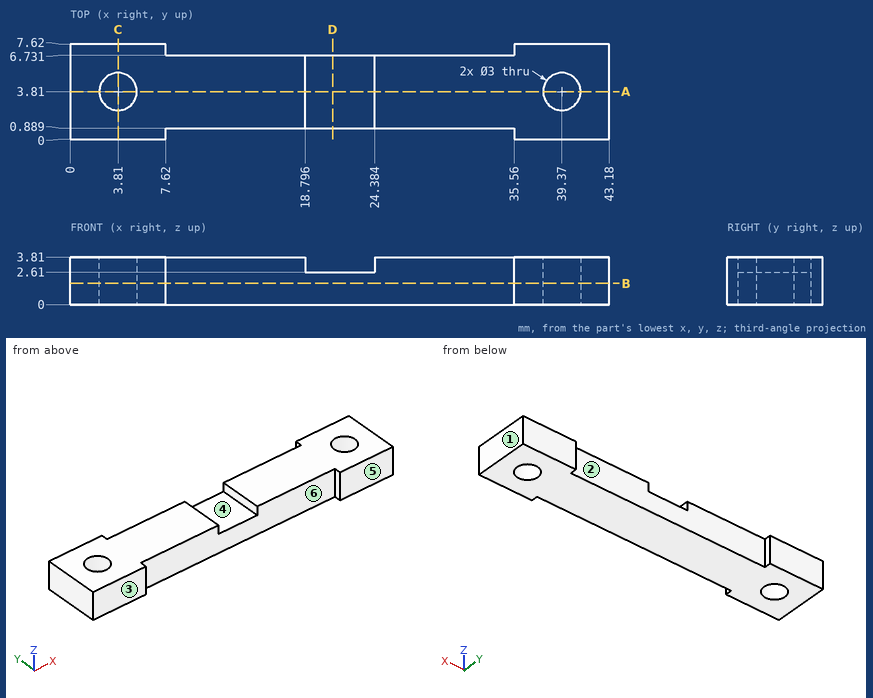
Answer from the drawing. Dimensions are ordinates in mm from the lowest x, y and z of the part. A direction names the side the tool comes from. Give positions to 0.01 mm unless a question says otherwise; leave off trailing zeros. Loops run counter-clockwise (first coordinate to the right, second up) from the corner with the lowest first, then second, coordinate; pieces in that order, holes last. Notation, with made-up numbers: (64, 80) - (96, 80) arc R20 ccw to (96, 113) - close; hole circle Ø7 at (86, 4). An arc over 180 degrees is marked (long way). Answer as CSV lines item,"result". Start each with the question number.
Item 1: Each of these flat-tipped pins is pushed along its axis until it touches: pin 1 (1.9 mm diameter, centred on x = 26, z = 1, fed in from +Y); pin 2 (2.5 mm diameter, centred on x = 3.81, y = 3.81, fed in from +Z). Where does it stop, or does it pass through?
Item 2: A cutting plane is placed at D-D on x = 21. Determine the outline of the cut face in (y, z).
Item 3: A cutting plane is placed at C-C on x = 3.81. Determine the outline of the cut face in (y, z).
Item 4: The mould has two halves that part along X. Classify the marked faces 1, 2, 3 and 4: +X half, -X half, draft (parallel to the pull), parting line (faces both ways), or undercut.
Item 5: A cutting plane is placed at A-A on y = 3.81. Determine the outline of the cut face in (x, z).
Item 6: For the marked faces 5 and 6, determine the directions among +Z, -Z, +X, -X, +Y, -Y from which every point of the face is accessible in a straight line to the end or side of a thin tool.
Item 7: Find the intervals of material crossed by line 1 (X direction, y = 3.81, z = 1.4); line 2 (X direction, y = 3.81, z = 2.7); line 3 (X direction, y = 0.75, z = 1.4), in increasing order. Write a range as from..to.
Item 8: A cutting plane is placed at B-B on z = 1.7. Determine the outline of the cut face in (x, y).
Found:
1,pin 1,"stops at y = 6.73"
1,pin 2,"passes through"
2,outline,"(0.89, 0) - (6.73, 0) - (6.73, 2.61) - (0.89, 2.61) - close"
3,outline,"(0, 0) - (2.31, 0) - (2.31, 3.81) - (0, 3.81) - close; (5.31, 0) - (7.62, 0) - (7.62, 3.81) - (5.31, 3.81) - close"
4,face 1,"+X half"
4,face 2,"undercut"
4,face 3,"draft"
4,face 4,"undercut"
5,outline,"(0, 0) - (2.31, 0) - (2.31, 3.81) - (0, 3.81) - close; (5.31, 0) - (37.87, 0) - (37.87, 3.81) - (24.38, 3.81) - (24.38, 2.61) - (18.8, 2.61) - (18.8, 3.81) - (5.31, 3.81) - close; (40.87, 0) - (43.18, 0) - (43.18, 3.81) - (40.87, 3.81) - close"
6,face 5,"+Z, -Z, +X, -X, -Y"
6,face 6,"+Z, -Z, -Y"
7,line 1,"x = 0..2.31, 5.31..37.87, 40.87..43.18"
7,line 2,"x = 0..2.31, 5.31..18.8, 24.38..37.87, 40.87..43.18"
7,line 3,"x = 0..7.62, 35.56..43.18"
8,outline,"(0, 0) - (7.62, 0) - (7.62, 0.89) - (35.56, 0.89) - (35.56, 0) - (43.18, 0) - (43.18, 7.62) - (35.56, 7.62) - (35.56, 6.73) - (7.62, 6.73) - (7.62, 7.62) - (0, 7.62) - close; hole circle Ø3 at (3.81, 3.81); hole circle Ø3 at (39.37, 3.81)"
